Check sheet for the modelled part. Datum: model origin and axes. Units: mm. A direction names the side the tool comes from. Coordinates: 2 decimals unless noted, no trailing zeros. Order: outer loops, then holes, each group sorted by start corner. A loop starts at its lowest first (then second) coordinate and runs counter-clockwise, first axis right, second up.
1. Set-up check for faces 1 (the flat face through (0, -6.35, -5)), 2 (the flat face through (-0.4, 6.5, -10)), 3 (the cylindrical face through (-22.415, -13.017, 14.79)): record each of +Z, -Z, +X, -X, +Y, -Y from which the full face is reachable in a straight line by a thin tool's end or side.
2. Cross-section at B-B (z = 21). Enter the section's corners in (x, y), then the cut area to 3 significant figures.
3. Cross-section at A-A (y = 0). Enter the section's corners in (x, z), then the cut area to 3 significant figures.
4. Gauge pin test, flat ends, axial feed: pin 1 Ø2 at (y, z) = (5.5, 1.5) entering from +X; pin 2 Ø10 at (x, z) = (21.5, 11) entering from -Y; pin 3 Ø4 at (y, z) = (-12.5, 20.5) entering from +X; pin 4 Ø2.5 at (x, y) = (-6.35, 6.35) entering from +Z. Record the tip position at first contact, or that the pin passes through.
5. Cross-section at D-D (y = -18.5). Enter the section's corners in (x, z), then the cut area to 3 significant figures.
6. Cross-section at C-C (x = -1). Enter the section's corners in (y, z).
7. Thickness scan on line 1 (Y direction, x = 0, z = 18); line 2 (Y direction, x = 21, z = 5); line 3 (Z direction, x = -9.5, y = 14.5). Record the ranges inside material, lowest first.
8. Draft check along X on faces 4 (the flat face through (-10.3, -18.2, 30)), 5 (the flat face through (10, 0, 0)). Enter one of: released by +X, released by -X, zero draft, split by the parting line, or undercut.
```python
from build123d import *

# Parameters (mm, degrees)
F0_R     = 27.5
F1_DEPTH = 10
F2_DEPTH = 30


with BuildPart() as f1:
    # F0 (on Top) → F1 (new body)
    with BuildSketch(Plane.XY):
        Circle(F0_R)
        with BuildLine():
            ThreePointArc((22.75, 11.8356805184), (22.0909902577, 10.2446902607), (20.5, 9.5856805184))
            Line((20.5, 9.5856805184), (20.5, -9.5856805184))
            ThreePointArc((20.5, -9.5856805184), (22.0909902577, -10.2446902607), (22.75, -11.8356805184))
            ThreePointArc((22.75, -11.8356805184), (21.0823428515, -14.0090136275), (18.5514428415, -12.9606805184))
            Line((18.5514428415, -12.9606805184), (1.9485571585, -22.5463610368))
            ThreePointArc((1.9485571585, -22.5463610368), (2.1733331092, -23.0890181853), (2.25, -23.6713610368))
            ThreePointArc((2.25, -23.6713610368), (-0.5823428515, -25.8446941459), (-1.9485571585, -22.5463610368))
            Line((-1.9485571585, -22.5463610368), (-18.5514428415, -12.9606805184))
            ThreePointArc((-18.5514428415, -12.9606805184), (-22.4485571585, -12.9606805184), (-20.5, -9.5856805184))
            Line((-20.5, -9.5856805184), (-20.5, 9.5856805184))
            ThreePointArc((-20.5, 9.5856805184), (-22.4485571585, 12.9606805184), (-18.5514428415, 12.9606805184))
            Line((-18.5514428415, 12.9606805184), (-1.9485571585, 22.5463610368))
            ThreePointArc((-1.9485571585, 22.5463610368), (-0.5823428515, 25.8446941459), (2.25, 23.6713610368))
            ThreePointArc((2.25, 23.6713610368), (2.1733331092, 23.0890181853), (1.9485571585, 22.5463610368))
            Line((1.9485571585, 22.5463610368), (18.5514428415, 12.9606805184))
            ThreePointArc((18.5514428415, 12.9606805184), (21.0823428515, 14.0090136275), (22.75, 11.8356805184))
        make_face(mode=Mode.SUBTRACT)
        with BuildLine():
            Line((20.5, -9.5856805184), (20.5, 9.5856805184))
            ThreePointArc((20.5, 9.5856805184), (18.5514428415, 10.7106805184), (18.5514428415, 12.9606805184))
            Line((18.5514428415, 12.9606805184), (1.9485571585, 22.5463610368))
            ThreePointArc((1.9485571585, 22.5463610368), (0, 21.4213610368), (-1.9485571585, 22.5463610368))
            Line((-1.9485571585, 22.5463610368), (-18.5514428415, 12.9606805184))
            ThreePointArc((-18.5514428415, 12.9606805184), (-18.3266668908, 12.4180233699), (-18.25, 11.8356805184))
            ThreePointArc((-18.25, 11.8356805184), (-18.9090097423, 10.2446902607), (-20.5, 9.5856805184))
            Line((-20.5, 9.5856805184), (-20.5, -9.5856805184))
            ThreePointArc((-20.5, -9.5856805184), (-18.9090097423, -10.2446902607), (-18.25, -11.8356805184))
            ThreePointArc((-18.25, -11.8356805184), (-18.3266668908, -12.4180233699), (-18.5514428415, -12.9606805184))
            Line((-18.5514428415, -12.9606805184), (-1.9485571585, -22.5463610368))
            ThreePointArc((-1.9485571585, -22.5463610368), (0, -21.4213610368), (1.9485571585, -22.5463610368))
            Line((1.9485571585, -22.5463610368), (18.5514428415, -12.9606805184))
            ThreePointArc((18.5514428415, -12.9606805184), (18.5514428415, -10.7106805184), (20.5, -9.5856805184))
        make_face()
        with BuildLine():
            ThreePointArc((-6.35, 4.85), (-7.4106601718, 7.4106601718), (-4.85, 6.35))
            Line((-4.85, 6.35), (4.85, 6.35))
            ThreePointArc((4.85, 6.35), (6.35, 7.85), (7.85, 6.35))
            ThreePointArc((7.85, 6.35), (7.4106601718, 5.2893398282), (6.35, 4.85))
            Line((6.35, 4.85), (6.35, -4.85))
            ThreePointArc((6.35, -4.85), (7.4106601718, -5.2893398282), (7.85, -6.35))
            ThreePointArc((7.85, -6.35), (6.35, -7.85), (4.85, -6.35))
            Line((4.85, -6.35), (-4.85, -6.35))
            ThreePointArc((-4.85, -6.35), (-7.4106601718, -7.4106601718), (-6.35, -4.85))
            Line((-6.35, -4.85), (-6.35, 4.85))
        make_face(mode=Mode.SUBTRACT)
        with BuildLine():
            Line((-20.5, 11.8356805184), (-18.5514428415, 12.9606805184))
            ThreePointArc((-18.5514428415, 12.9606805184), (-22.4485571585, 12.9606805184), (-20.5, 9.5856805184))
            Line((-20.5, 9.5856805184), (-20.5, 11.8356805184))
        make_face()
        with BuildLine():
            ThreePointArc((-20.5, -9.5856805184), (-22.4485571585, -12.9606805184), (-18.5514428415, -12.9606805184))
            Line((-18.5514428415, -12.9606805184), (-20.5, -11.8356805184))
            Line((-20.5, -11.8356805184), (-20.5, -9.5856805184))
        make_face()
        with BuildLine():
            Line((0, 23.6713610368), (1.9485571585, 22.5463610368))
            ThreePointArc((1.9485571585, 22.5463610368), (2.1733331092, 23.0890181853), (2.25, 23.6713610368))
            ThreePointArc((2.25, 23.6713610368), (-0.5823428515, 25.8446941459), (-1.9485571585, 22.5463610368))
            Line((-1.9485571585, 22.5463610368), (0, 23.6713610368))
        make_face()
        with BuildLine():
            Line((18.5514428415, 12.9606805184), (20.5, 11.8356805184))
            Line((20.5, 11.8356805184), (20.5, 9.5856805184))
            ThreePointArc((20.5, 9.5856805184), (22.0909902577, 10.2446902607), (22.75, 11.8356805184))
            ThreePointArc((22.75, 11.8356805184), (21.0823428515, 14.0090136275), (18.5514428415, 12.9606805184))
        make_face()
        with BuildLine():
            ThreePointArc((22.75, -11.8356805184), (22.0909902577, -10.2446902607), (20.5, -9.5856805184))
            Line((20.5, -9.5856805184), (20.5, -11.8356805184))
            Line((20.5, -11.8356805184), (18.5514428415, -12.9606805184))
            ThreePointArc((18.5514428415, -12.9606805184), (21.0823428515, -14.0090136275), (22.75, -11.8356805184))
        make_face()
        with BuildLine():
            ThreePointArc((2.25, -23.6713610368), (2.1733331092, -23.0890181853), (1.9485571585, -22.5463610368))
            Line((1.9485571585, -22.5463610368), (0, -23.6713610368))
            Line((0, -23.6713610368), (-1.9485571585, -22.5463610368))
            ThreePointArc((-1.9485571585, -22.5463610368), (-0.5823428515, -25.8446941459), (2.25, -23.6713610368))
        make_face()
        with BuildLine():
            Line((-20.5, -11.8356805184), (-18.5514428415, -12.9606805184))
            ThreePointArc((-18.5514428415, -12.9606805184), (-18.3266668908, -12.4180233699), (-18.25, -11.8356805184))
            ThreePointArc((-18.25, -11.8356805184), (-18.9090097423, -10.2446902607), (-20.5, -9.5856805184))
            Line((-20.5, -9.5856805184), (-20.5, -11.8356805184))
        make_face()
        with BuildLine():
            ThreePointArc((-18.25, 11.8356805184), (-18.3266668908, 12.4180233699), (-18.5514428415, 12.9606805184))
            Line((-18.5514428415, 12.9606805184), (-20.5, 11.8356805184))
            Line((-20.5, 11.8356805184), (-20.5, 9.5856805184))
            ThreePointArc((-20.5, 9.5856805184), (-18.9090097423, 10.2446902607), (-18.25, 11.8356805184))
        make_face()
        with BuildLine():
            ThreePointArc((-1.9485571585, 22.5463610368), (0, 21.4213610368), (1.9485571585, 22.5463610368))
            Line((1.9485571585, 22.5463610368), (0, 23.6713610368))
            Line((0, 23.6713610368), (-1.9485571585, 22.5463610368))
        make_face()
        with BuildLine():
            Line((20.5, 9.5856805184), (20.5, 11.8356805184))
            Line((20.5, 11.8356805184), (18.5514428415, 12.9606805184))
            ThreePointArc((18.5514428415, 12.9606805184), (18.5514428415, 10.7106805184), (20.5, 9.5856805184))
        make_face()
        with BuildLine():
            Line((20.5, -11.8356805184), (20.5, -9.5856805184))
            ThreePointArc((20.5, -9.5856805184), (18.5514428415, -10.7106805184), (18.5514428415, -12.9606805184))
            Line((18.5514428415, -12.9606805184), (20.5, -11.8356805184))
        make_face()
        with BuildLine():
            Line((0, -23.6713610368), (1.9485571585, -22.5463610368))
            ThreePointArc((1.9485571585, -22.5463610368), (0, -21.4213610368), (-1.9485571585, -22.5463610368))
            Line((-1.9485571585, -22.5463610368), (0, -23.6713610368))
        make_face()
    extrude(amount=-F1_DEPTH)

    # F0 (on Top) → F2 (join)
    with BuildSketch(Plane.XY):
        Circle(F0_R)
        with BuildLine():
            ThreePointArc((22.75, 11.8356805184), (22.0909902577, 10.2446902607), (20.5, 9.5856805184))
            Line((20.5, 9.5856805184), (20.5, -9.5856805184))
            ThreePointArc((20.5, -9.5856805184), (22.0909902577, -10.2446902607), (22.75, -11.8356805184))
            ThreePointArc((22.75, -11.8356805184), (21.0823428515, -14.0090136275), (18.5514428415, -12.9606805184))
            Line((18.5514428415, -12.9606805184), (1.9485571585, -22.5463610368))
            ThreePointArc((1.9485571585, -22.5463610368), (2.1733331092, -23.0890181853), (2.25, -23.6713610368))
            ThreePointArc((2.25, -23.6713610368), (-0.5823428515, -25.8446941459), (-1.9485571585, -22.5463610368))
            Line((-1.9485571585, -22.5463610368), (-18.5514428415, -12.9606805184))
            ThreePointArc((-18.5514428415, -12.9606805184), (-22.4485571585, -12.9606805184), (-20.5, -9.5856805184))
            Line((-20.5, -9.5856805184), (-20.5, 9.5856805184))
            ThreePointArc((-20.5, 9.5856805184), (-22.4485571585, 12.9606805184), (-18.5514428415, 12.9606805184))
            Line((-18.5514428415, 12.9606805184), (-1.9485571585, 22.5463610368))
            ThreePointArc((-1.9485571585, 22.5463610368), (-0.5823428515, 25.8446941459), (2.25, 23.6713610368))
            ThreePointArc((2.25, 23.6713610368), (2.1733331092, 23.0890181853), (1.9485571585, 22.5463610368))
            Line((1.9485571585, 22.5463610368), (18.5514428415, 12.9606805184))
            ThreePointArc((18.5514428415, 12.9606805184), (21.0823428515, 14.0090136275), (22.75, 11.8356805184))
        make_face(mode=Mode.SUBTRACT)
    extrude(amount=F2_DEPTH)


solid = f1.part
```
Data:
1. face 1: +Z, -Z
1. face 2: -Z, +X, -X, +Y, -Y
1. face 3: +Z
2. outline: circle Ø55 at (0, 0); hole (-20.5, -9.59) arc R2.25 ccw (long way) to (-18.55, -12.96) - (-1.95, -22.55) arc R2.25 ccw (long way) to (1.95, -22.55) - (18.55, -12.96) arc R2.25 ccw (long way) to (20.5, -9.59) - (20.5, 9.59) arc R2.25 ccw (long way) to (18.55, 12.96) - (1.95, 22.55) arc R2.25 ccw (long way) to (-1.95, 22.55) - (-18.55, 12.96) arc R2.25 ccw (long way) to (-20.5, 9.59) - close
2. area: 856 mm2
3. outline: (-27.5, -10) - (-6.35, -10) - (-6.35, 0) - (-20.5, 0) - (-20.5, 30) - (-27.5, 30) - close; (6.35, -10) - (27.5, -10) - (27.5, 30) - (20.5, 30) - (20.5, 0) - (6.35, 0) - close
3. area: 843 mm2
4. pin 1: stops at x = 27.13
4. pin 2: stops at y = -22
4. pin 3: stops at x = 25.42
4. pin 4: passes through
5. outline: (-20.35, -10) - (20.35, -10) - (20.35, 30) - (8.96, 30) - (8.96, 0) - (-8.96, 0) - (-8.96, 30) - (-20.35, 30) - close
5. area: 1,090 mm2
6. outline: (-27.48, -10) - (-6.35, -10) - (-6.35, 0) - (-25.69, 0) - (-25.69, 30) - (-27.48, 30) - close; (6.35, -10) - (27.48, -10) - (27.48, 30) - (25.69, 30) - (25.69, 0) - (6.35, 0) - close
7. line 1: y = -27.5 to -25.92, 25.92 to 27.5
7. line 2: y = -17.76 to -14.03, -9.64 to 9.64, 14.03 to 17.76
7. line 3: z = -10 to 0
8. face 4: zero draft
8. face 5: undercut
